Autodesk Inventor part; units mm, degrees
ref_plane "YZ Plane" through (0, 0, 0) normal (1, 0, 0) x (0, 1, 0)
ref_plane "XZ Plane" through (0, 0, 0) normal (0, 1, 0) x (-1, 0, 0)
ref_plane "XY Plane" through (0, 0, 0) normal (0, 0, 1) x (1, 0, 0)
ref_plane "Work Plane1" through (0, 0, 0) normal (0, 0, 1) x (1, 0, 0)
sketch "Sketch1" plane through (0, 0, 0) normal (0, 0, 1) x (1, 0, 0)
  line L0 (28, 30) -> (30, 28) construction
  line L1 (28, 30) -> (-28, 30) construction
  line L2 (-30, 28) -> (-28, 30) construction
  line L3 (-30, 28) -> (-30, -28) construction
  line L4 (-28, -30) -> (-30, -28) construction
  line L5 (-28, -30) -> (28, -30) construction
  line L6 (30, -28) -> (28, -30) construction
  line L7 (30, -28) -> (30, 28) construction
  circle A0 centre (-17.5, -17.5) radius 1.95
  circle A1 centre (17.5, 17.5) radius 1.95
  circle A2 centre (17.5, -17.5) radius 1.95
  circle A3 centre (-17.5, 17.5) radius 1.95
  circle A4 centre (0, 0) radius 7.5 construction
  line L8 (-52.85, 44) -> (87.15, 44) construction
  line L9 (-30, -30) -> (30, -30)
  line L10 (30, -30) -> (30, 44)
  line L11 (30, 44) -> (-30, 44)
  line L12 (-30, 44) -> (-30, -30)
  line L13 (42.65, -13) -> (79.65, -13) construction
  line L14 (42.65, 36.7) -> (42.65, -13) construction
  line L15 (79.65, 36.7) -> (42.65, 36.7) construction
  line L16 (79.65, 36.7) -> (79.65, -13) construction
  line L17 (79.65, -13) -> (30, -13)
  line L18 (30, -13) -> (30, 23.9)
  line L19 (30, 23.9) -> (79.65, 23.9)
  line L20 (79.65, 23.9) -> (79.65, -13)
  line L21 (-15, -15) -> (15, -15)
  line L22 (15, -15) -> (15, 15)
  line L23 (15, 15) -> (-15, 15)
  line L24 (-15, 15) -> (-15, -15)
  line L25 (-15, -15) -> (15, 15) construction
  line L26 (15, -15) -> (-15, 15) construction
  circle A5 centre (48.55, -3.3) radius 4.5
  circle A6 centre (61.15, 21.7) radius 4.5
  circle A7 centre (73.75, -3.3) radius 4.5
  line L27 (25, -25) -> (-25, -25) construction
  line L28 (-25, -25) -> (-25, 25) construction
  line L29 (-25, 25) -> (25, 25) construction
  line L30 (25, 25) -> (25, -25) construction
  line L31 (25, -25) -> (-25, 25) construction
  line L32 (-25, -25) -> (25, 25) construction
  circle A8 centre (-25, 25) radius 1.75
  circle A9 centre (25, 25) radius 1.75
  circle A10 centre (25, -25) radius 1.75
  circle A11 centre (-25, -25) radius 1.75
  point P0 (0, 0)
  dimension "d6" = 30
  dimension "d7" = 30
  dimension "d57" = 50
  dimension "d58" = 50
  dimension "d59" = 3.5
  dimension "d60" = 3.5
  dimension "d61" = 3.5
  dimension "d62" = 3.5
extrude "Extrusion1" add sketch "Sketch1" along normal blind 8 contours A0 | A1 | A2 | A3 | L12 L11 L10 L9 | L10 L19 A6 L20 L17 | L19 A6 | A5 | A7 picked at (60.9501, 21.68)
sketch "Sketch2" plane through (-30, 44, 0) normal (0, 1, 0) x (1, 0, 0)
  line L0 (60, 0) -> (60, -8)
  line L1 (0, 0) -> (0, -8)
  line L2 (60, -8) -> (0, -8)
  circle A0 centre (88.9869, -30.1976) radius 1.4 construction
  circle A1 centre (91.15, -56.0499) radius 15 construction
  line L3 (0, -8) -> (70, -8)
  line L4 (70, -8) -> (70, -68)
  line L5 (70, -68) -> (0, -68)
  line L6 (0, -68) -> (0, -8)
  point P0 (30, 0)
  dimension "d2" = 70
  dimension "d3" = 60
extrude "Extrusion2" add sketch "Sketch2" against normal blind 8
sketch "Sketch3" plane through (0, 0, 8) normal (0, 0, 1) x (1, 0, 0)
  line L0 (30, 36) -> (-30, 36)
  line L1 (-30, 36) -> (-30, -30)
  line L2 (-30, -30) -> (30, -30)
  line L3 (30, -30) -> (30, -13)
  line L4 (30, -13) -> (79.65, -13)
  line L5 (79.65, -13) -> (79.65, 23.9)
  line L6 (79.65, 23.9) -> (30, 23.9)
  line L7 (30, 23.9) -> (30, 36)
  point P0 (0, 0)
sketch "Sketch4" plane through (-30, -30, 0) normal (-1, 0, 0) x (0, 0, 1)
  line L0 (0, 74) -> (0, 0)
  line L1 (0, 0) -> (8, 0)
  line L2 (8, 66) -> (8, 0)
  line L3 (68, 66) -> (8, 66)
  line L4 (68, 74) -> (68, 66)
  line L5 (0, 74) -> (68, 74)
  line L6 (68, 66) -> (8, 7.9065)
  line L7 (8, 53.9) -> (8, 66)
  line L8 (8, 7.9065) -> (8, 66)
  line L9 (8, 66) -> (68, 66)
  line L10 (8, 66) -> (68, 66)
  point P0 (0, 30)
extrude "Extrusion3" add sketch "Sketch4" against normal blind 4
pattern_linear "Rectangular Pattern1" count 2 spacing 56 along (1, 0, 0) of "Extrusion3"
sketch "Sketch7" plane through (30, 23.9, 0) normal (0, 1, 0) x (1, 0, 0)
  arc A0 (57.15, -64.5499) -> (60.65, -61.0499) centre (57.15, -61.0499) ccw
  line L0 (60.65, -2.1699) -> (60.65, -61.0499)
  arc A1 (60.65, -2.1699) -> (57.15, 1.3301) centre (57.15, -2.1699) ccw
  line L1 (-82.85, 1.3301) -> (57.15, 1.3301)
  arc A2 (-82.85, 1.3301) -> (-86.35, -2.1699) centre (-82.85, -2.1699) ccw
  line L2 (-86.35, -61.0499) -> (-86.35, -2.1699)
  arc A3 (-86.35, -61.0499) -> (-82.85, -64.5499) centre (-82.85, -61.0499) ccw
  line L3 (57.15, -64.5499) -> (-82.85, -64.5499)
  line L4 (49.65, 0) -> (49.65, -8)
  line L5 (49.65, -8) -> (39.65, -8)
  line L6 (39.65, -8) -> (39.65, -38)
  line L7 (39.65, -38) -> (49.65, -38) construction
  line L8 (49.65, -38) -> (49.65, -8)
  arc A4 (39.65, -38) -> (49.65, -38) centre (44.65, -38) ccw
  circle A5 centre (44.65, -38) radius 1.55
  point P0 (-30, 0)
  dimension "d25" = 10
  dimension "d26" = 30
  dimension "d27" = 3.1
extrude "Extrusion5" add sketch "Sketch7" along normal up to surface (57 mm away) from surface at -36.9 contours L8 A4 L6 L5
fillet "Fillet1" radius 10 1 edges at (69.65, 5.45, 8)
sketch "Sketch8" plane through (79.65, -13, 0) normal (1, 0, 0) x (0, 0, -1)
  line L0 (0, 0) -> (0, 36.9)
  line L1 (0, 36.9) -> (-8, 36.9)
  line L2 (-38, 0) -> (-38, 57)
  line L3 (0, 0) -> (-38, 0)
  line L4 (-38, 36.9) -> (-43, 36.9)
  line L5 (-43, 36.9) -> (-33, 36.9)
  line L6 (-33, 36.9) -> (-33, 31.9)
  line L7 (-33, 31.9) -> (-43, 31.9)
  line L8 (-43, 31.9) -> (-43, 36.9)
  line L9 (-8, 57) -> (-8, 36.9)
  line L10 (-8, 57) -> (-38, 57)
  point P0 (0, 13)
  dimension "d31" = 10
  dimension "d32" = 5
extrude "Extrusion6" cut sketch "Sketch8" against normal up to surface (10 mm away) contours L7 L8 L4 L2 | L2 L5 L6 L7
pattern_linear "Rectangular Pattern2" count 6 spacing 10 along (0, -1, 0) count 3 spacing 10 along (0, 1, 0) of "Extrusion6"
sketch "Sketch9" plane through (0, 0, 0) normal (0, 0, -1) x (-1, 0, 0)
  line L0 (15, 15) -> (15, -15)
  line L1 (15, -15) -> (-15, -15)
  line L2 (-15, -15) -> (-15, 15)
  line L3 (-15, 15) -> (15, 15)
  line L4 (-79.65, -13) -> (-79.65, 23.9)
  line L5 (-30, -13) -> (-79.65, -13)
  line L6 (30, -30) -> (-30, -30)
  line L7 (30, 44) -> (30, -30)
  line L8 (-30, 44) -> (30, 44)
  line L9 (-79.65, 23.9) -> (-30, 23.9)
  circle A0 centre (-61.2, 5.45) radius 18.45 construction
  circle A1 centre (-61.2, 5.45) radius 6.3
  line L10 (-30, 23.9) -> (-30, 44)
  line L11 (-30, -30) -> (-30, -13)
  point P0 (0, 0)
  dimension "d38" = 12.6
extrude "Extrusion7" cut sketch "Sketch9" against normal blind 10 contours A1
sketch "Sketch10" plane through (0, 0, 8) normal (0, 0, 1) x (1, 0, 0)
  circle A0 centre (61.2, 5.45) radius 6.3
  circle A1 centre (61.2, 5.45) radius 10.3
  point P0 (0, 0)
  dimension "d47" = 4
extrude "Extrusion8" add sketch "Sketch10" along normal blind 4
sketch "Sketch12" plane through (-30, 44, 0) normal (0, 1, 0) x (1, 0, 0)
  line L0 (60, 0) -> (0, 0)
  line L1 (0, 0) -> (0, -68)
  line L2 (70, -68) -> (0, -68)
  line L3 (70, -8) -> (70, -68)
  line L4 (60, -8) -> (70, -8)
  line L5 (60, 0) -> (60, -8)
  circle A0 centre (35, -33) radius 35
  line L6 (50, -58) -> (10, -58) construction
  line L7 (10, -58) -> (10, -18) construction
  line L8 (10, -18) -> (50, -18) construction
  line L9 (50, -18) -> (50, -58) construction
  line L10 (50, -58) -> (10, -18) construction
  line L11 (10, -58) -> (50, -18) construction
  point P0 (30, 0)
  point P1 (30, -38)
  dimension "d48" = 40
  dimension "d49" = 40
hole "Hole2" at (-20, 44, 58) at (-20, 44, 18) at (20, 44, 58) at (20, 44, 18) direction (0, -1, 0) diameter 2.8 end through all
sketch "Sketch13" plane through (0, 0, 8) normal (0, 0, 1) x (1, 0, 0)
  arc A0 (-26, -26.4361) -> (-26, -23.5639) centre (-25, -25) ccw
  arc A1 (-26, 23.5639) -> (-26, 26.4361) centre (-25, 25) ccw
  arc A2 (26, 26.4361) -> (26, 23.5639) centre (25, 25) ccw
  arc A3 (26, -23.5639) -> (26, -26.4361) centre (25, -25) ccw
  point P0 (0, 0)
hole "Hole3" at (-25, -25, 8) at (-25, 25, 8) at (25, 25, 8) at (25, -25, 8) direction (0, 0, -1) diameter 3.9 depth 10 tip angle 118
sketch "Sketch14" plane through (0, 0, 8) normal (0, 0, 1) x (1, 0, 0)
  arc A0 (26, 26.6741) -> (26, 23.3259) centre (25, 25) ccw
  line L0 (26, 26.6741) -> (26, 36)
  line L1 (26, 36) -> (-26, 36)
  line L2 (-26, 36) -> (-26, 26.6741)
  arc A1 (-26, 23.3259) -> (-26, 26.6741) centre (-25, 25) ccw
  line L3 (-26, 23.3259) -> (-26, -22.0935)
  line L4 (-26, -22.0935) -> (-30, -22.0935)
  line L5 (-30, -22.0935) -> (-30, -30)
  line L6 (-30, -30) -> (30, -30)
  line L7 (30, -30) -> (30, -22.0935)
  line L8 (30, -22.0935) -> (26, -22.0935)
  line L9 (26, -22.0935) -> (26, 23.3259)
  circle A2 centre (-25, -25) radius 1.95
  circle A3 centre (25, -25) radius 1.95
  line L10 (-15, -15) -> (-15, 15)
  line L11 (-15, 15) -> (15, 15)
  line L12 (15, 15) -> (15, -15)
  line L13 (15, -15) -> (-15, -15)
  circle A4 centre (-25, 25) radius 4
  arc A5 (26, 26.6741) -> (26, 23.3259) centre (25, 25) ccw
  circle A6 centre (25, 25) radius 4
  point P0 (0, 0)
  dimension "d70" = 8
  dimension "d71" = 8
extrude "Extrusion10" cut sketch "Sketch14" along normal blind 14 contours L0 A6 L9 A0 | A0 L9 A6 L0 | A4 L3 A1 L2 | L2 A1 L3 A4
sketch "Sketch15" plane through (30, 23.9, 0) normal (0, 1, 0) x (1, 0, 0)
  line L0 (49.65, 0) -> (49.65, -8)
  line L1 (49.65, 0) -> (0, 0)
  line L2 (0, -8) -> (0, 0)
  line L3 (29.65, -8) -> (0, -8)
  arc A0 (39.65, -18) -> (29.65, -8) centre (29.65, -18) ccw
  line L4 (39.65, -8) -> (39.65, -18)
  line L5 (49.65, -8) -> (39.65, -8)
  point P0 (-30, 0)
extrude "Extrusion11" add sketch "Sketch15" along normal up to surface (20.1 mm away)
sketch "Sketch16" plane through (-30, 44, 0) normal (0, 1, 0) x (1, 0, 0)
  line L0 (109.65, -33) -> (99.65, -33)
  line L1 (70, -8) -> (70, -68)
  line L2 (0, 0) -> (109.65, 0)
  line L3 (109.65, -33) -> (70, -33)
  line L4 (70, -33) -> (70, 0)
  line L5 (70, 0) -> (109.65, 0)
  line L6 (109.65, 0) -> (109.65, -33)
  point P0 (30, 0)
extrude "Extrusion12" add sketch "Sketch16" against normal blind 5
sketch "Sketch17" plane through (79.65, -13, 0) normal (1, 0, 0) x (0, 0, -1)
  line L0 (-33, 56.9) -> (-33, 51.9)
  line L1 (-33, 51.9) -> (-38, 51.9)
  line L2 (-38, 46.9) -> (-38, 51.9)
  line L3 (-38, 46.9) -> (-33, 46.9)
  line L4 (-33, 46.9) -> (-33, 41.9)
  line L5 (-33, 41.9) -> (-38, 41.9)
  line L6 (-38, 36.9) -> (-38, 41.9)
  line L7 (-38, 36.9) -> (-33, 36.9)
  line L8 (-33, 36.9) -> (-33, 31.9)
  line L9 (-33, 31.9) -> (-38, 31.9)
  line L10 (-38, 26.9) -> (-38, 31.9)
  line L11 (-38, 26.9) -> (-33, 26.9)
  line L12 (-33, 26.9) -> (-33, 21.9)
  line L13 (-33, 21.9) -> (-38, 21.9)
  line L14 (-38, 16.9) -> (-38, 21.9)
  line L15 (-38, 16.9) -> (-33, 16.9)
  line L16 (-33, 16.9) -> (-33, 11.9)
  line L17 (-33, 11.9) -> (-38, 11.9)
  line L18 (-38, 6.9) -> (-38, 11.9)
  line L19 (-38, 6.9) -> (-33, 6.9)
  line L20 (-33, 6.9) -> (-33, 1.9)
  line L21 (-33, 1.9) -> (-38, 1.9)
  line L22 (-38, 0) -> (-38, 1.9)
  line L23 (0, 0) -> (-38, 0)
  line L24 (0, 0) -> (0, 57)
  line L25 (0, 57) -> (-38, 57)
  line L26 (-38, 56.9) -> (-38, 57)
  line L27 (-38, 56.9) -> (-33, 56.9)
  line L28 (-33, 56.9) -> (-33, 51.9)
  line L29 (-33, 51.9) -> (-38, 51.9)
  line L30 (-38, 51.9) -> (-38, 57.6693)
  line L31 (-38, 57.6693) -> (-33, 57.6693)
  line L32 (-33, 57.6693) -> (-33, 51.9)
  line L33 (-32.2207, 6.9) -> (-43.7781, 6.9)
  line L34 (-43.7781, 6.9) -> (-43.7781, -2.7729)
  line L35 (-43.7781, -2.7729) -> (-32.2207, -2.7729)
  line L36 (-32.2207, -2.7729) -> (-32.2207, 6.9)
  line L37 (-33, 51.9) -> (-45.418, 51.9)
  line L38 (-45.418, 51.9) -> (-45.418, 59.4654)
  line L39 (-45.418, 59.4654) -> (-33, 59.4654)
  line L40 (-33, 59.4654) -> (-33, 51.9)
  point P0 (0, 13)
extrude "Extrusion13" cut sketch "Sketch17" against normal up to surface (10 mm away) contours L0 L1 L30 L27 | L27 L26 L25 L32 | L30 L37 L38 L39 L40 L31 L26 | L25 L30 L31 L32 | L36 L35 L34 L33 L19 L20 L21 L22 L23 | L23 L22 L21 L20 L33 L36
properties part number "cellSTORM_cellphone_objectivelens_mount"
Design review of the part built by this model. Coordinates are the model's own, in mm. A direction names the side the tool comes from. Round coordinates to 2 decimals unless told otherwise and drop trailing zeros. Write each loop counter-clockwise with the first axis right and the second up, starting at its lowest first coordinate (ties: lowest second). Pieces come first, ordered by that corner, then holes. Notation, with made-up numbers: M -19,33.5 L -14,33.5 A27 cw -14,71.5 Z; hole C 8,59 d8. An arc over 180 degrees is marked long. One line per item, written item: value. Start each with the question number.
1. Clearance check with flat-ended pins moving along their axes: P1, Ø4, axis at x = 7, z = 31.5, coming from the -Y side; P2, Ø2.5, axis at x = 25, y = 25, coming from the -Z side; P3, Ø4, axis at x = 74.5, y = 30, coming from the +Z side. State where each tip first meets the part, or that it passes through.
2. Take a section at B-B on z = 58. State the section outline as (x, y) points, then the cut area to 3 significant figures.
3. Take a section at A-A on y = 5.45. State the section outline as (x, z) points, then the cut area to 3 significant figures.
4. Take a section at C-C on x = 36. State the section outline as (y, z) points, then the cut area to 3 significant figures.
5. For faces 1 (the face through (-15, 0, 4)), 2 (the face through (75, 13.9, 36)), 3 (the face through (26, 14, 31)), 4 (the face through (75, 38.9, 36)), 5 (the face through (66, -13, 9)), list the 3-axis set-ups (+Z, -Z, +X, -X, +Y, -Y) from which the entire face can be reached by the end or side of a thin tool; tool diameter is ignored.
6. Draft analysis for pull direction X (two halves, no side actions). For faces 6 (the face through (75, 21, 33)), 7 (the face through (-19.46, 39.94, 59.29)), state which applies: pulls with the +X half, pulls with the -X half, needs draft (parallel to the pull), parting line crosses it, or undercut.
7. To check wall thickness, follow probe 1 along Y at (x, z) = (-25, 2); probe 2 along X at (y, z) = (-3.5, 19.5); probe 3 along X at (y, z) = (39, 58). State the ranges of each line that lie inside material, in increasing order. Write a range as from..to.
8. Take a section at D-D on x = 74.65. State how many separate pieces and enclosed holes the cut face has, then the cut area to 3 significant figures.
Computed:
1. P1: stops at y = 36
1. P2: stops at z = 22
1. P3: stops at z = 43
2. outline: M -30,26.32 L -26,26.32 L -26,36 L -21.4,36 L -21.4,44 L -30,44 Z; M -18.6,36 L 18.6,36 L 18.6,44 L -18.6,44 Z; M 21.4,36 L 26,36 L 26,26.32 L 30,26.32 L 30,36 L 40,36 L 40,44 L 21.4,44 Z
2. area: 593 mm²
3. outline: M -30,0 L -15,0 L -15,8 L -26,8 L -26,36.45 L -30,36.45 Z; M 15,0 L 54.9,0 L 54.9,12 L 50.9,12 L 50.9,8 L 30,8 L 30,36.45 L 26,36.45 L 26,8 L 15,8 Z; M 65.65,10 L 67.5,10 L 67.5,0 L 79.65,0 L 79.65,38 A5 ccw 69.65,38 L 69.65,18 A10 cw 67.65,12 L 67.5,12 L 67.5,11.81 A10 cw Z; hole C 74.65,38 d3.1
3. area: 1,130 mm²
4. outline: M -13,0 L 44,0 L 44,68 L 36,68 L 36,8 L -13,8 Z
4. area: 936 mm²
5. face 1: +Z, -Z
5. face 2: +Z, +X
5. face 3: +Z, -Y
5. face 4: +Z, +X, +Y
5. face 5: +Z, -Z, +X, -Y
6. face 6: needs draft
6. face 7: undercut
7. probe 1: y = -30..-26.95, -23.05..23.05, 26.95..44
7. probe 2: x = -30..-26, 26..30, 69.65..79.65
7. probe 3: x = -30..-21.4, -18.6..18.6, 21.4..40
8. separate pieces: 6
8. enclosed holes: 0
8. area: 2,050 mm²
